Input: part model. Units: mm. Frame: model coordinates. Face numbers are marked on the shaded views. A direction names the side the tool comes from. Round coordinates to 2 decimals unless told otherwise and drop trailing zeros. Loops run counter-clockwise (first coordinate to the right, second up) from the corner with the lowest first, then second, coordinate; pieces in that order, holes last. Notation, with made-up numbers: M 29.25,16.5 L 45.25,16.5 A19 ccw 45.25,33.5 Z; hole C 39,-2 d4. An arc over 180 degrees is marked long. Use one line per item in the form item = value. Start each with the question number.
Q1. Ray query, line 1 along Z through (x, y) = (-0.25, -0.25); line 2 along Z through (x, y) = (-3.45, -0.1); line 3 along X through (y, z) = (0.1, 10.25). Return the intervals inside material, ascending.
Q2. Section query A-A, the plane y = 0.9. Output: boundary loops of the cut face in (x, z), and give its area (3 significant figures).
Q3. Section query C-C, the plane z = 11.25. Output: boundary loops of the cut face in (x, y).
Q4. Access query for the marked faces 1, 2 and 3. Directions: +Z, -Z, +X, -X, +Y, -Y. A direction counts if a zero-diameter tool reaches every point of the face in a straight line with its end or side. Return the directions, or none.
Q5. Section query D-D, the plane x = -3.4. Output: boundary loops of the cut face in (y, z), and give its area (3 significant figures).
Q6. Section query B-B, the plane x = -0.45. Output: boundary loops of the cut face in (y, z), and give its area (3 significant figures).
Q7. First-contact query: P1, Ø1.5, axis at x = 0, y = -0.5, coming from the +Z side; P2, Ø1.5, axis at x = -0.5, z = 9.5, coming from the +Y side. Flat tips, straight axial feed; report the tip coordinate or a pass-through.
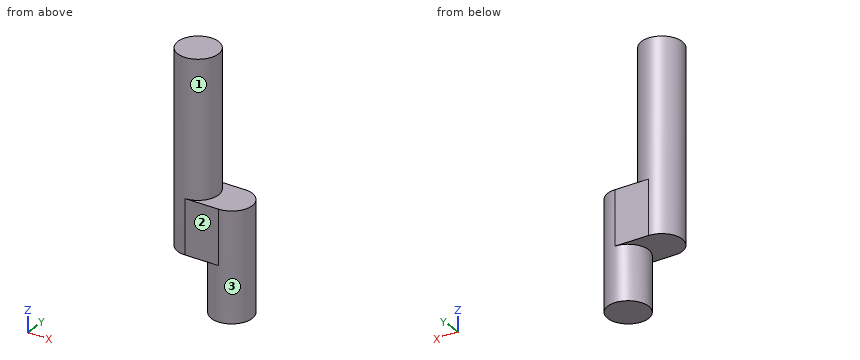
Autodesk Inventor part; units mm, degrees
ref_plane "YZ Plane" through (0, 0, 0) normal (1, 0, 0) x (0, 1, 0)
ref_plane "XZ Plane" through (0, 0, 0) normal (0, 1, 0) x (-1, 0, 0)
ref_plane "XY Plane" through (0, 0, 0) normal (0, 0, 1) x (1, 0, 0)
sketch "草图1" plane through (0, 0, 0) normal (0, 0, 1) x (1, 0, 0)
  circle A0 centre (0, 0) radius 1.5
  dimension "d0" = 3
extrude "拉伸1" add sketch "草图1" along normal blind 4
sketch "草图2" plane through (0, 0, 4) normal (0, 0, 1) x (1, 0, 0)
  arc A0 (0, -1.5) -> (0, 1.5) centre (0, 0) ccw
  circle A1 centre (0, 0) radius 1.5
  line L0 (0, -1.5) -> (-2.5, -1.5)
  line L1 (0, 1.5) -> (-2.5, 1.5)
  line L2 (-2.5, 1.5) -> (-2.5, -1.5)
  arc A2 (-2.5, 1.5) -> (-2.5, -1.5) centre (-2.5, 0) ccw
  dimension "d3" = 2.5
extrude "拉伸2" add sketch "草图2" along normal blind 4
sketch "草图3" plane through (0, 0, 8) normal (0, 0, 1) x (1, 0, 0)
  arc A0 (-2.5, 1.5) -> (-2.5, -1.5) centre (-2.5, 0) ccw
  circle A1 centre (-2.5, 0) radius 1.5
  point P0 (0, 0)
extrude "拉伸3" add sketch "草图3" along normal blind 10
properties part number "偏心支轴"
Results found:
q1.line_1 = 0 to 8
q1.line_2 = 4 to 18
q1.line_3 = -4 to -1
q2.outline = M -3.7,4 L -1.2,4 L -1.2,0 L 1.2,0 L 1.2,8 L -1.3,8 L -1.3,18 L -3.7,18 Z
q2.area = 53.2 mm²
q3.outline = C -2.5,0 d3
q4.face_1 = +Z
q4.face_2 = +Z, -Z, +X, -X, -Y
q4.face_3 = -Z
q5.outline = M -1.2,4 L 1.2,4 L 1.2,18 L -1.2,18 Z
q5.area = 33.6 mm²
q6.outline = M -1.5,4 L -1.43,4 L -1.43,0 L 1.43,0 L 1.43,4 L 1.5,4 L 1.5,8 L -1.5,8 Z
q6.area = 23.4 mm²
q7.P1 = 8
q7.P2 = 0.83
